Verification items for the finished model (mm, model axes). Face numbers are marked on the shaded views. A direction names the side the tool comes from. Round coordinates to 2 decimals unless told otherwise and drop trailing zeros. Loops run counter-clockwise (first coordinate to the right, second up) from the corner with the lowest first, then second, coordinate; pieces in that order, holes last.
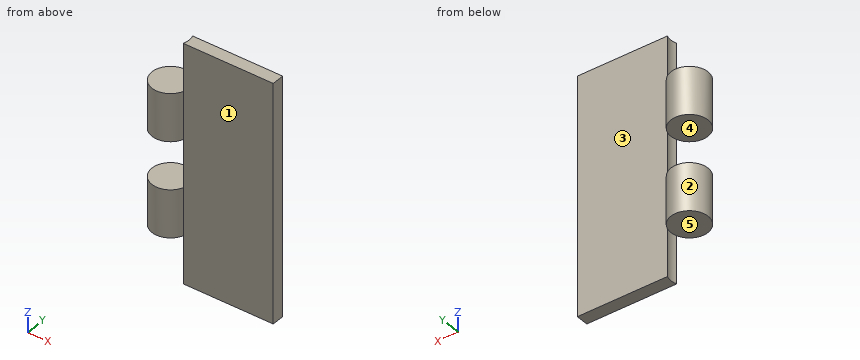
from build123d import *

# Parameters (mm, degrees)
BOSS_EXTRUDE1_DEPTH = 101.6
SKETCH1_3_R         = 7.9375
CUT_EXTRUDE1_DEPTH  = 20.32
CUT_EXTRUDE2_START  = 60.96
SKETCH1_5_R         = 7.9375
CUT_EXTRUDE2_DEPTH  = 20.32
CUT_EXTRUDE3_START  = 81.28
SKETCH1_6_R         = 7.9375
CUT_EXTRUDE3_DEPTH  = 20.32


with BuildPart() as part:
    # Sketch1 → Boss-Extrude1 (new body)
    with BuildSketch(Plane.XY):
        with BuildLine():
            Line((7.476029511, -2.667), (46.0375, -2.667))
            Line((46.0375, -2.667), (46.0375, 2.667))
            Line((46.0375, 2.667), (7.476029511, 2.667))
            ThreePointArc((7.476029511, 2.667), (-7.9375, 0), (7.476029511, -2.667))
        make_face()
    extrude(amount=BOSS_EXTRUDE1_DEPTH)

    # Sketch1_3 → Cut-Extrude1 (cut)
    with BuildSketch(Plane.XY):
        Circle(SKETCH1_3_R)
    extrude(amount=CUT_EXTRUDE1_DEPTH, mode=Mode.SUBTRACT)

    # Sketch1_5 → Cut-Extrude2 (cut)
    with BuildSketch(Plane.XY.offset(CUT_EXTRUDE2_START)):
        Circle(SKETCH1_5_R)
    extrude(amount=-CUT_EXTRUDE2_DEPTH, mode=Mode.SUBTRACT)

    # Sketch1_6 → Cut-Extrude3 (cut)
    with BuildSketch(Plane.XY.offset(CUT_EXTRUDE3_START)):
        Circle(SKETCH1_6_R)
    extrude(amount=CUT_EXTRUDE3_DEPTH, mode=Mode.SUBTRACT)


solid = part.part
1. Gauge pin test, flat ends, axial feed: P1, Ø5, axis at x = 32, z = 66.5, coming from the +Y side; P2, Ø8, axis at x = 9.5, z = 60, coming from the +Y side; P3, Ø3, axis at y = 5, z = 23, coming from the +X side. Record the tip position at first contact, or that the pin passes through.
2. Scan lines: L1, parallel to Y at x = 35, z = 90.5; L2, parallel to Z at x = -4, y = 4; L3, parallel to X at y = 0, z = 5.5. Record each from-to range of solid material in increasing order.
3. Tool access check on the marked faces 1 and 2. Record the directions out of +Z, -Z, +X, -X, +Y, -Y that give a thin tool (end or side, any length) a straight path to the whole face; none if there is none.
4. Release check for a two-part mould opening along Z. For the marked faces 3, 4 and 5 record: released by +Z, released by -Z, zero draft, split by the parting line, or undercut.
5. Section check A-A (x = 0). Enter the section's corners in (y, z).
6. Section check B-B (y = 0). Enter the section's corners in (x, z), then the cut area to 3 significant figures.
7. Section check C-C (y = -5.75). Enter the section's corners in (x, z), then the cut area to 3 significant figures.
8. Section check D-D (x = 22.5). Enter the section's corners in (y, z).
Taken from the geometry:
1. P1: stops at y = 2.67
1. P2: stops at y = 5.61
1. P3: stops at x = 7.12
2. L1: y = -2.67 to 2.67
2. L2: z = 20.32 to 40.64, 60.96 to 81.28
2. L3: x = 7.94 to 46.04
3. face 1: +Z, -Z, +X, -Y
3. face 2: +Z, -Z
4. face 3: zero draft
4. face 4: undercut
4. face 5: released by -Z
5. outline: (-7.94, 20.32) - (7.94, 20.32) - (7.94, 40.64) - (-7.94, 40.64) - close; (-7.94, 60.96) - (7.94, 60.96) - (7.94, 81.28) - (-7.94, 81.28) - close
6. outline: (-7.94, 20.32) - (7.94, 20.32) - (7.94, 0) - (46.04, 0) - (46.04, 101.6) - (7.94, 101.6) - (7.94, 81.28) - (-7.94, 81.28) - (-7.94, 60.96) - (7.94, 60.96) - (7.94, 40.64) - (-7.94, 40.64) - close
6. area: 4,520 mm2
7. outline: (-5.47, 20.32) - (5.47, 20.32) - (5.47, 40.64) - (-5.47, 40.64) - close; (-5.47, 60.96) - (5.47, 60.96) - (5.47, 81.28) - (-5.47, 81.28) - close
7. area: 445 mm2
8. outline: (-2.67, 0) - (2.67, 0) - (2.67, 101.6) - (-2.67, 101.6) - close
